The listing builds one solid part. Answer for the finished solid, in the listing's coordinates (mm). A direction names the side the tool comes from. Give positions to 0.01 mm unless a question says otherwise; leave off trailing zeros. Write each loop counter-clockwise with the first axis right and the second up, starting at its lowest first coordinate (ties: lowest second). Pieces come first, ordered by that corner, then holes. Notation, with made-up numbers: (-23.75, -3.5) -> (13.25, -3.5) arc R23 cw to (13.25, 26.5) -> close; hole circle Ø7 at (85, 47.25). An arc over 180 degrees is marked (long way). Write each question's results on one line, items separated by ' | '. Start each with the question number.
from build123d import *

# Parameters (mm, degrees)
SKETCH_1_W      = 23
SKETCH_1_H      = 10
EXTRUDE_1_DEPTH = 7.4
SKETCH_2_R      = 1.1
EXTRUDE_2_DEPTH = 1.6


with BuildPart() as part:
    # 草图1 → 凸台-拉伸1 (new body)
    with BuildSketch(Plane.XY):
        Rectangle(SKETCH_1_W, SKETCH_1_H)
    extrude(amount=EXTRUDE_1_DEPTH)

    # 草图2 → 凸台-拉伸2 (add)
    with BuildSketch(Plane(origin=(0, 0, 0), x_dir=(-1, 0, 0), z_dir=(0, 0, -1))):
        Polygon((-11.3, -2), (-11.3, -5.5), (11.3, -5.5), (11.3, -2), (15, -2), (15, 2), (11.3, 2), (11.3, 5.5), (-11.3, 5.5), (-11.3, 2), (-15, 2), (-15, -2), align=None)
        with Locations((-13, 0)):
            Circle(SKETCH_2_R, mode=Mode.SUBTRACT)
        with Locations((13, 0)):
            Circle(SKETCH_2_R, mode=Mode.SUBTRACT)
    extrude(amount=EXTRUDE_2_DEPTH)


solid = part.part
1. Consider probe 1 along Y at (x, z) = (13, -1.1); probe 2 along Y at (x, z) = (5, 5); probe 3 along X at (y, z) = (-2, 7). Determine where each line is inside the solid, lowest interval first. Write a range as [from, to].
2. Each of these flat-tipped pins is pushed along its axis until it touches: pin 1 Ø2 at (y, z) = (-0.5, 1.5) entering from -X; pin 2 Ø0.8 at (y, z) = (-3.5, -0.5) entering from +X; pin 3 Ø1.3 at (x, z) = (-13.5, -1) entering from -Y. Where does it stop, or does it pass through?
3. Section A-A (x = -13) is taken. Write down the section's boundary in (y, z), then the cut area to 3 significant figures.
4. Section C-C (x = 0.75) is taken. Write down the section's boundary in (y, z), then the cut area to 3 significant figures.
5. Section D-D (y = 3.75) is taken. Write down the section's boundary in (x, z), then the cut area to 3 significant figures.
6. Section B-B (y = 0) is taken. Write down the section's boundary in (x, z), then the cut area to 3 significant figures.
7. A tool of negligible diameter and unlimited length cuts with its end or side. For faces 1 (the flat face through (0, 5, 4)), 2 (the flat face through (14, 1, 0)), 3 (the flat face through (-11.5, 0, 4)), from which of +Z, -Z, +X, -X, +Y, -Y can it reach the whole face along a straight path? Write none if from no direction.
Results:
1) probe 1: y = [-2, -1.1], [1.1, 2] | probe 2: y = [-5, 5] | probe 3: x = [-11.5, 11.5]
2) pin 1: stops at x = -11.5 | pin 2: stops at x = 11.3 | pin 3: stops at y = -2
3) outline: (-2, -1.6) -> (-1.1, -1.6) -> (-1.1, 0) -> (-2, 0) -> close; (1.1, -1.6) -> (2, -1.6) -> (2, 0) -> (1.1, 0) -> close | area: 2.88 mm²
4) outline: (-5.5, -1.6) -> (5.5, -1.6) -> (5.5, 0) -> (5, 0) -> (5, 7.4) -> (-5, 7.4) -> (-5, 0) -> (-5.5, 0) -> close | area: 91.6 mm²
5) outline: (-11.5, 0) -> (-11.3, 0) -> (-11.3, -1.6) -> (11.3, -1.6) -> (11.3, 0) -> (11.5, 0) -> (11.5, 7.4) -> (-11.5, 7.4) -> close | area: 206 mm²
6) outline: (-15, -1.6) -> (-14.1, -1.6) -> (-14.1, 0) -> (-15, 0) -> close; (-11.9, -1.6) -> (11.9, -1.6) -> (11.9, 0) -> (11.5, 0) -> (11.5, 7.4) -> (-11.5, 7.4) -> (-11.5, 0) -> (-11.9, 0) -> close; (14.1, -1.6) -> (15, -1.6) -> (15, 0) -> (14.1, 0) -> close | area: 211 mm²
7) face 1: +Z, +X, -X, +Y | face 2: +Z, +X, +Y, -Y | face 3: +Z, -X, +Y, -Y
